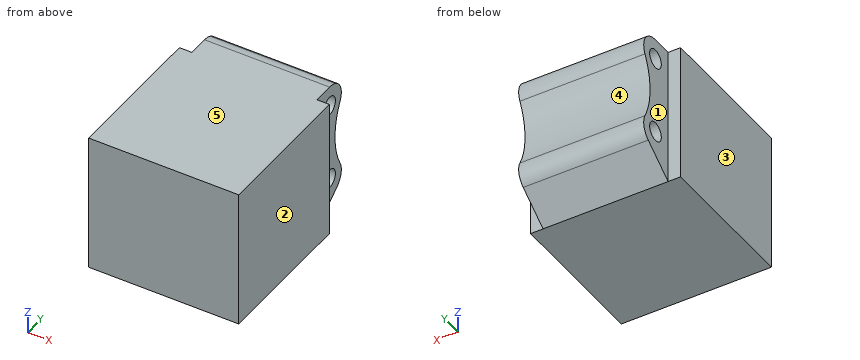
Autodesk Inventor part; units mm, degrees
ref_plane "YZ Plane" through (0, 0, 0) normal (1, 0, 0) x (0, 1, 0)
ref_plane "XZ Plane" through (0, 0, 0) normal (0, 1, 0) x (-1, 0, 0)
ref_plane "XY Plane" through (0, 0, 0) normal (0, 0, 1) x (1, 0, 0)
sketch "Sketch1" plane through (0, 0, 0) normal (1, 0, 0) x (0, 1, 0)
  circle A0 centre (-9.7574, -19.7073) radius 1.55 construction
  circle A1 centre (0, 0) radius 1.55 construction
  circle A2 centre (-9.7574, -19.7073) radius 2.65
  circle A3 centre (0, 0) radius 2.65
  line L0 (-6.0684, -24.2876) -> (12.7398, 12.1607) construction
  arc A4 (-12.2239, -24.4871) -> (-4.9776, -22.1738) centre (-9.7574, -19.7073) ccw
  circle A5 centre (0, 0) radius 5.7448
  line L1 (-4.9776, -22.1738) -> (5.1052, -2.6344)
  arc A6 (-4.9776, -22.1738) -> (-12.2239, -24.4871) centre (-9.7574, -19.7073) ccw
  line L2 (-14.5372, -17.2408) -> (-5.1904, 2.4623)
  line L3 (0, 0) -> (0, -27.0135) construction
  line L4 (0, 0) -> (-9.7574, -19.7073) construction
  point P0 (-10.1101, -25.5779)
  dimension "d0" = 5.3
  dimension "d1" = 5.3
  dimension "d3" = 11.4897
  dimension "d4" = 5.3787
  dimension "d5" = 21.8076
  dimension "d6" = 21.9875
extrude "Extrusion1" [suppressed]
sketch "Sketch4" plane through (0, 0, 0) normal (1, 0, 0) x (0, 1, 0)
  circle A0 centre (0, 0) radius 2.65
  circle A1 centre (0, 0) radius 5.7448
  line L0 (5.7448, 0) -> (5.7448, -21.991)
  line L1 (0, 0) -> (-9.7574, -19.7073) construction
  line L2 (5.7448, -21.991) -> (0, -21.991) construction
  circle A2 centre (0, -21.991) radius 5.7448
  circle A3 centre (0, -21.991) radius 2.65
  line L3 (-5.7448, -21.991) -> (-5.7448, 0)
  dimension "d22" = 21.991
  dimension "d23" = 21.9905
  dimension "d24" = 5.3
extrude "Extrusion4" add sketch "Sketch4" along normal mid plane 35
sketch "Sketch6" plane through (0, 0, 0) normal (1, 0, 0) x (0, 1, 0)
  line L0 (5.7448, 0) -> (5.7448, -21.991) construction
  arc A0 (-5.7448, -21.991) -> (5.7448, -21.991) centre (0, -21.991) ccw construction
  line L1 (-5.7448, -21.991) -> (-5.7448, 0) construction
  arc A1 (5.7448, 0) -> (-5.7448, 0) centre (0, 0) ccw construction
  circle A2 centre (0, -21.991) radius 2.65 construction
  circle A3 centre (0, 0) radius 2.65 construction
  arc A4 (5.7448, 0) -> (-5.7448, 0) centre (0, 0) ccw construction
  line L2 (0, 0) -> (-5.7448, 0) construction
  line L3 (0, 5.7448) -> (-5.7448, 5.7448) construction
  line L4 (-5.7448, 5.7448) -> (-5.7448, -33.2552) construction
  line L5 (-5.7448, 5.7448) -> (-46.9448, 5.7448) construction
  line L6 (-5.7448, -33.2552) -> (-46.9448, -33.2552)
  line L7 (-46.9448, -33.2552) -> (-46.9448, 5.7448)
  line L8 (-46.9448, 5.7448) -> (-5.7448, 5.7448)
  line L9 (-5.7448, 5.7448) -> (-5.7448, -33.2552)
  dimension "d32" = 39
  dimension "d35" = 41.2
extrude "Extrusion5" add sketch "Sketch6" along normal mid plane 42
sketch "Sketch7" plane through (17.5, 0, 0) normal (1, 0, 0) x (0, 0, -1)
  line L0 (21.991, 5.7448) -> (0, 5.7448)
  arc A0 (0, 5.7448) -> (0, -5.7448) centre (0, 0) ccw
  line L1 (0, -5.7448) -> (21.991, -5.7448)
  arc A1 (21.991, -5.7448) -> (21.991, 5.7448) centre (21.991, 0) ccw
  circle A2 centre (21.991, 0) radius 2.65
  circle A3 centre (0, 0) radius 2.65
  line L2 (-5.7448, -46.9448) -> (33.2552, -46.9448)
  line L3 (33.2552, -46.9448) -> (33.2552, -5.7448)
  line L4 (33.2552, -5.7448) -> (-5.7448, -5.7448)
  line L5 (-5.7448, -5.7448) -> (-5.7448, -46.9448)
  line L6 (33.2552, -5.7448) -> (26.6413, 3.3732)
  arc A4 (21.991, -5.7448) -> (21.991, 5.7448) centre (21.991, 0) ccw
  line L7 (-5.7448, -5.7448) -> (-5.7448, 0)
  arc A5 (0, 5.7448) -> (0, -5.7448) centre (0, 0) ccw
  point P0 (26.6413, 3.3732)
  point P1 (0, -5.7448)
extrude "Extrusion6" add sketch "Sketch7" against normal up to surface (35 mm away) contours A1 L1 A0 L0 | L6 L4 A1 | A0 L4 L7
sketch "Sketch8" plane through (17.5, 0, 0) normal (1, 0, 0) x (0, 0, -1)
  line L0 (21.991, 5.7448) -> (0, 5.7448)
  arc A0 (0, 5.7448) -> (-5.7448, 0) centre (0, 0) ccw
  line L1 (-5.7448, 0) -> (-5.7448, -5.7448)
  line L2 (33.2552, -5.7448) -> (-5.7448, -5.7448)
  line L3 (33.2552, -5.7448) -> (26.6413, 3.3732)
  arc A1 (26.6413, 3.3732) -> (21.991, 5.7448) centre (21.991, 0) ccw
  circle A2 centre (21.991, 0) radius 2.65
  circle A3 centre (0, 0) radius 2.65
  line L4 (0, 5.7448) -> (21.991, 5.7448)
  arc A4 (26.6413, 3.3732) -> (21.991, 5.7448) centre (21.991, 0) ccw
  arc A5 (0, 5.7448) -> (21.991, 5.7448) centre (10.9955, 22.4511) ccw
  dimension "d39" = 20
extrude "Extrusion7" cut sketch "Sketch8" against normal up to next contours A5 L0
fillet "Fillet1" radius 5 2 edges at (0, 5.7448, -21.991) (0, 5.7448, 0)
properties part number "Kauri modular session 5 mount" material "Brass, Soft Yellow"
Geometry: final body of the model. Coordinates: model frame, mm. Face numbers are marked on the shaded views. A direction names the side the tool comes from. Give positions to 0.01 mm unless a question says otherwise; leave off trailing zeros. Loops run counter-clockwise (first coordinate to the right, second up) from the corner with the lowest first, then second, coordinate; pieces in that order, holes last. Notation, with made-up numbers: M 73.5,29.25 L 78.5,29.25 A31 cw 78.5,66.25 Z; hole C -1,67.5 d2. An arc over 180 degrees is marked long. Put each result on its own line as item: value.
1) First-contact query: P1, Ø12, axis at y = 1.5, z = -16.5, coming from the +X side; P2, Ø9, axis at y = -1, z = -11, coming from the -X side; P3, Ø1, axis at x = -19, z = -19, coming from the +Y side; P4, Ø8, axis at x = 9, y = -2, coming from the -Z side. Flat tips, straight axial feed; report the tip coordinate or a pass-through.
Computed values:
P1: stops at x = 17.5
P2: stops at x = -17.5
P3: stops at y = -5.74
P4: stops at z = -33.26
2) Cut plane B-B, the plane x = 13.5. Give the number of separate pieces and of enclosed holes in the cut face, plus the area to 3 significant figures.
Computed values:
separate pieces: 1
enclosed holes: 2
area: 1,900 mm^2
3) Cut plane A-A, the plane z = -9. Return the cut outline in (x, y).
Computed values:
outline: M -21,-46.94 L 21,-46.94 L 21,-5.74 L 17.5,-5.74 L 17.5,2.55 L -17.5,2.55 L -17.5,-5.74 L -21,-5.74 Z
4) Material intervals for L1, parallel to Z at x = 3, y = 0; L2, parallel to Z at x = -2, y = 2; L3, parallel to Y at x = 1.5, z = 0, sorted ascending. Write a range as from..to.
Computed values:
L1: z = -29.09..-24.64, -19.34..-2.65, 2.65..5.74
L2: z = -27.64..-23.73, -20.25..-1.74, 1.74..5.39
L3: y = -46.94..-2.65, 2.65..5.29
5) Reachability of the marked faces 1 and 2 from +Z, -Z, +X, -X, +Y, -Y: full face, straight path, thin tool, end or side. Return the list, or none.
Computed values:
face 1: +Z, -Z, -X, +Y
face 2: +Z, -Z, +X, +Y, -Y
6) Mould query, pull axis Z, two halves, no side actions, for the marked faces 3, 4 and 5. Classes: released by +Z, released by -Z, zero draft, split by the parting line, or undercut.
Computed values:
face 3: zero draft
face 4: undercut
face 5: released by +Z
7) Cut plane C-C, the plane z = -15. Return the cut outline in (x, y), plus the area to 3 significant figures.
Computed values:
outline: M -21,-46.94 L 21,-46.94 L 21,-5.74 L 17.5,-5.74 L 17.5,2.86 L -17.5,2.86 L -17.5,-5.74 L -21,-5.74 Z
area: 2,030 mm^2
